For this review, take the finished solid that the model builds, in its own axes (mm). Face numbers are marked on the shaded views. A direction names the side the tool comes from. Give positions to 0.01 mm unless a question says otherwise; leave off trailing zeros. Loops run counter-clockwise (first coordinate to the right, second up) from the corner with the lowest first, then second, coordinate; pieces in that order, holes last.
```python
from build123d import *


with BuildPart() as part:
    # Croquis1 → Revolución1 (revolve)
    with BuildSketch(Plane(origin=(0, 0, 0), x_dir=(0, 0, -1), z_dir=(1, 0, 0)), mode=Mode.PRIVATE) as revoluci_n1_sk:
        Polygon((2, 3), (-23, 3), (-23, 9), (-19, 9), (-19, 13), (-15, 13), (-15, 21), (-13, 21), (-13, 31), (0, 31), (0, 30), (-11, 27), (-11, 10), (2, 10), align=None)
    revolve(revoluci_n1_sk.sketch.rotate(Axis((0, 0, 0), (0, 0, 1)), 90), axis=Axis((0, 0, 0), (0, 0, 1)))


solid = part.part
```
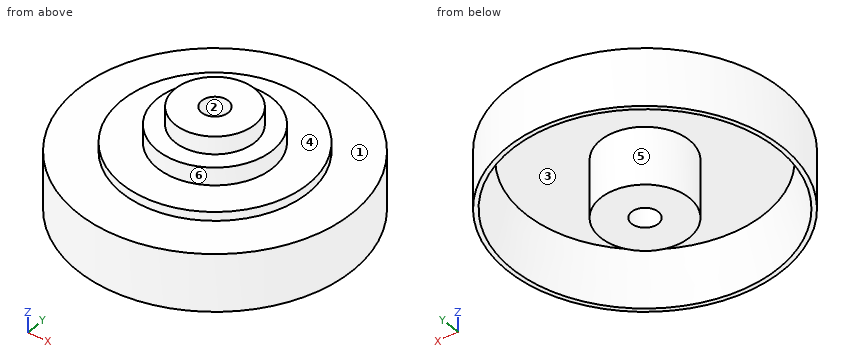
Q1. Mouldability with a two-part tool opening along X and no side actions: class the marked faces 4, 5 and 6 as +X half, -X half, draft (parallel to the pull), parting line (faces both ways), or undercut.
Answers:
face 4: draft
face 5: undercut
face 6: parting line
Q2. Consider section C-C on z = 8.75. Give the boundary of the cut face in (x, y).
Answers:
outline: circle Ø62 at (0, 0); circle Ø20 at (0, 0); hole circle Ø55.23 at (0, 0); hole circle Ø6 at (0, 0)
Q3. Machinability: for the marked faces 1, 2 and 3, which of the approach directions +Z, -Z, +X, -X, +Y, -Y give a long, thin tool a straight path to every point of the face, cutting with its end or side? Answer none if there is none.
Answers:
face 1: +Z
face 2: +Z, -Z
face 3: -Z
Q4. For probe 1 along Y at (x, z) = (0, 7.75); probe 2 along Z at (x, y) = (14.5, 18.5); probe 3 along Y at (x, z) = (25, 6.5), list the stretches that pass through material, from the lowest coordinate up.
Answers:
probe 1: y = -31 to -27.89, -10 to -3, 3 to 10, 27.89 to 31
probe 2: z = 11 to 13
probe 3: y = -18.33 to -13.11, 13.11 to 18.33
Q5. Consider section A-A on y = 0. Give the boundary of the cut face in (x, z).
Answers:
outline: (-31, 0) - (-30, 0) - (-27, 11) - (-10, 11) - (-10, -2) - (-3, -2) - (-3, 23) - (-9, 23) - (-9, 19) - (-13, 19) - (-13, 15) - (-21, 15) - (-21, 13) - (-31, 13) - close; (3, -2) - (10, -2) - (10, 11) - (27, 11) - (30, 0) - (31, 0) - (31, 13) - (21, 13) - (21, 15) - (13, 15) - (13, 19) - (9, 19) - (9, 23) - (3, 23) - close
Q6. For pin 1 Ø1 at (x, y) = (13.5, -9.5) entering from +Z; pin 2 Ø5 at (x, y) = (0, 0) entering from -Z; pin 3 Ø5 at (x, z) = (-22, 7.5) entering from +Y; pin 4 Ø8 at (x, z) = (11, 8) entering from +Y, all flat-tipped, find the tip position at first contact; note any pin that passes through.
Answers:
pin 1: stops at z = 15
pin 2: passes through
pin 3: stops at y = 24.1
pin 4: stops at y = 30.2
